The listing builds one solid part. Answer for the finished solid, in the listing's coordinates (mm). Round coordinates to 2 decimals unless told otherwise and drop trailing zeros. Write each loop counter-clockwise with the first axis right and the second up, starting at its lowest first coordinate (ties: lowest second). Pieces come first, ordered by that corner, then holes.
Item 1: Find the intervals of material crossed by probe 1 along Y at (x, z) = (22.5, 0.8); probe 2 along X at (y, z) = (-23.5, 0.3), in increasing order.
Item 2: Find section C-C on z = 1.35. Give the number of separate pieces and of enclosed holes in the cut face, then the cut area to 3 significant figures.
Item 3: Find section B-B on y = -22.5. Give the vertices of the cut face in (x, z), then the cut area to 3 significant figures.
Item 4: Find section A-A on x = 22.5. Give the vertices of the cut face in (y, z), then the cut area to 3 significant figures.
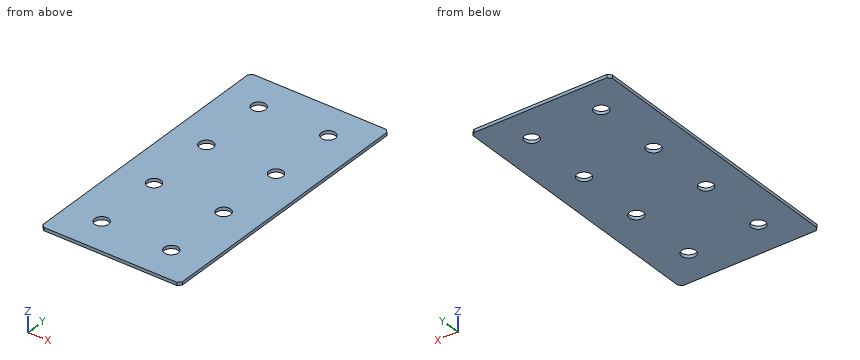
```python
from build123d import *

# Parameters (mm, degrees)
SKETCH_1_W        = 90
SKETCH_1_H        = 180
EXTRUDE_1_DEPTH   = 2
CHAMFER_1_SIZE    = 2
HOLE_WIZARD_M81_D = 9


with BuildPart() as part:
    # Эскиз1 → Бобышка-Вытянуть1 (new body)
    with BuildSketch(Plane.XY):
        Rectangle(SKETCH_1_W, SKETCH_1_H)
    extrude(amount=EXTRUDE_1_DEPTH)

    # Фаска1
    chamfer_1_edges = [part.edges().sort_by_distance(p)[0] for p in [
        (45, -90, 1),
        (-45, -90, 1),
        (-45, 90, 1),
        (45, 90, 1),
    ]]
    chamfer(chamfer_1_edges, length=CHAMFER_1_SIZE)

    # Отверстие с зазором M81 (through all)
    with Locations(Plane.XY.offset(2)):
        with Locations((-22.5, 22.5), (22.5, 22.5), (-22.5, -22.5), (22.5, -22.5), (-22.5, 67.5), (22.5, 67.5), (22.5, -67.5), (-22.5, -67.5)):
            Hole(HOLE_WIZARD_M81_D / 2)


solid = part.part
```
Check values:
1. probe 1: y = -90 to -72, -63 to -27, -18 to 18, 27 to 63, 72 to 90
1. probe 2: x = -45 to -26.89, -18.11 to 18.11, 26.89 to 45
2. separate pieces: 1
2. enclosed holes: 8
2. area: 15,700 mm2
3. outline: (-45, 0) - (-27, 0) - (-27, 2) - (-45, 2) - close; (-18, 0) - (18, 0) - (18, 2) - (-18, 2) - close; (27, 0) - (45, 0) - (45, 2) - (27, 2) - close
3. area: 144 mm2
4. outline: (-90, 0) - (-72, 0) - (-72, 2) - (-90, 2) - close; (-63, 0) - (-27, 0) - (-27, 2) - (-63, 2) - close; (-18, 0) - (18, 0) - (18, 2) - (-18, 2) - close; (27, 0) - (63, 0) - (63, 2) - (27, 2) - close; (72, 0) - (90, 0) - (90, 2) - (72, 2) - close
4. area: 288 mm2
